from build123d import *

# Parameters (mm, degrees)
SKETCH1_W           = 36.2
SKETCH1_H           = 29.5
BOSS_EXTRUDE1_DEPTH = 5
SKETCH3_W           = 33.053
SKETCH3_H           = 12.372
CUT_EXTRUDE1_DEPTH  = 47.964774033
SKETCH4_W           = 5
SKETCH4_H           = 12.372
BOSS_EXTRUDE2_DEPTH = 3.5
SKETCH5_R           = 14.763665
SKETCH5_R_2         = 12.2036
BOSS_EXTRUDE3_DEPTH = 10


with BuildPart() as part:
    # Sketch1 → Boss-Extrude1 (new body)
    with BuildSketch(Plane.XY):
        with Locations((18.1, 14.75)):
            Rectangle(SKETCH1_W, SKETCH1_H)
    extrude(amount=BOSS_EXTRUDE1_DEPTH)

    # Sketch3 → Cut-Extrude1 (cut, through all)
    with BuildSketch(Plane.XY.offset(5)):
        with Locations((18.1, 14.914)):
            Rectangle(SKETCH3_W, SKETCH3_H)
    extrude(amount=-CUT_EXTRUDE1_DEPTH, mode=Mode.SUBTRACT)

    # Sketch4 → Boss-Extrude2 (add)
    with BuildSketch(Plane.XY.offset(5)):
        with Locations((4.0735, 14.914)):
            Rectangle(SKETCH4_W, SKETCH4_H)
        with Locations((32.1265, 14.914)):
            Rectangle(SKETCH4_W, SKETCH4_H)
    extrude(amount=-BOSS_EXTRUDE2_DEPTH)

    # Sketch5 → Boss-Extrude3 (add)
    with BuildSketch(Plane.XY.offset(5)):
        with Locations(Location((23.79465, 14.75, 0), (0, 0, 204.072563575))):
            Circle(SKETCH5_R)
        with Locations(Location((23.79465, 14.75, 0), (0, 0, 209.568314483))):
            Circle(SKETCH5_R_2, mode=Mode.SUBTRACT)
    extrude(amount=BOSS_EXTRUDE3_DEPTH)


solid = part.part
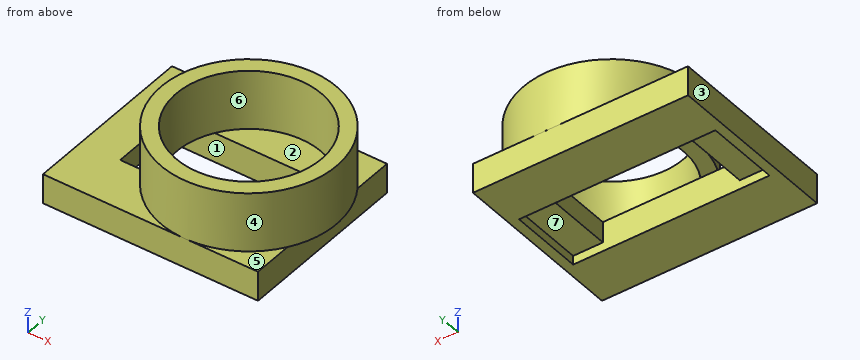
Geometry: final body of the model. Coordinates: model frame, mm. Face numbers are marked on the shaded views. A direction names the side the tool comes from. Give positions to 0.01 mm unless a question says otherwise; leave off trailing zeros. Write each loop counter-clockwise with the first axis right and the second up, starting at its lowest first coordinate (ties: lowest second). Pieces come first, ordered by that corner, then holes. Notation, with made-up numbers: (47.25, 81) - (68.25, 81) arc R20 ccw to (68.25, 104) - close; hole circle Ø9 at (36.5, 17). An arc over 180 degrees is marked (long way). Return JSON: item names as keys, results as strings. Group by question number.
1) Section C-C on y = 7.25. Return the cut outline in (x, z), plus the area to 3 significant figures.
2) First-contact query: P1, Ø3, axis at y = 16.5, z = 4, coming from the +X side; P2, Ø1.3, axis at x = 11.5, y = 12.5, coming from the -Z side; P3, Ø8, axis at y = 15, z = 13, coming from the -X side. Flat tips, straight axial feed; report the tip coordinate or a pass-through.
3) Section D-D on x = 31. Return the cut outline in (y, z).
4) Section B-B on y = 14.75. Return the cut outline in (x, z).
5) Line query: line 1 (X direction, y = 14.75, z = 11.75); line 2 (Y direction, x = 7.5, z = 1.25); line 3 (Y direction, x = 24, z = 13). Output: solid intervals per line, ascending.
6) Mould query, pull axis Y, two halves, no side actions, for the marked faces 1, 2, 3 and 4. Classes: released by +Y, released by -Y, zero draft, split by the parting line, or undercut.
7) Set-up query: the marked faces 5, 6 and 7. Return all of +Z, -Z, +X, -X, +Y, -Y with unobstructed straight access to the full face (end or side cutting, diameter ignored); none if empty.
8) Section A-A on x = 26.5. Return the cut outline in (y, z).
Filled in:
{
 "1": {"outline": "(0, 0) - (36.2, 0) - (36.2, 5) - (36.51, 5) - (36.51, 15) - (33.42, 15) - (33.42, 5) - (14.17, 5) - (14.17, 15) - (11.08, 15) - (11.08, 5) - (0, 5) - close", "area": "243 mm^2"},
 "2": {"P1": "stops at x = 38.54", "P2": "stops at z = 5", "P3": "stops at x = 9.03"},
 "3": {"outline": "(0, 0) - (8.73, 0) - (8.73, 1.5) - (21.1, 1.5) - (21.1, 0) - (29.5, 0) - (29.5, 5) - (27.64, 5) - (27.64, 15) - (24.6, 15) - (24.6, 5) - (4.9, 5) - (4.9, 15) - (1.86, 15) - (1.86, 5) - (0, 5) - close"},
 "4": {"outline": "(0, 0) - (1.57, 0) - (1.57, 1.5) - (6.57, 1.5) - (6.57, 5) - (0, 5) - close; (9.03, 5) - (11.59, 5) - (11.59, 15) - (9.03, 15) - close; (29.63, 1.5) - (34.63, 1.5) - (34.63, 0) - (36.2, 0) - (36.2, 5) - (38.56, 5) - (38.56, 15) - (36, 15) - (36, 5) - (29.63, 5) - close"},
 "5": {"line 1": "x = 9.03 to 11.59, 36 to 38.56", "line 2": "y = 0 to 8.73, 21.1 to 29.5", "line 3": "y = -0.01 to 2.55, 26.95 to 29.51"},
 "6": {"face 1": "undercut", "face 2": "undercut", "face 3": "zero draft", "face 4": "split by the parting line"},
 "7": {"face 5": "+Z, +X, -Y", "face 6": "+Z", "face 7": "-Z"},
 "8": {"outline": "(0, 0) - (8.73, 0) - (8.73, 5) - (2.85, 5) - (2.85, 15) - (0.24, 15) - (0.24, 5) - (0, 5) - close; (21.1, 0) - (29.5, 0) - (29.5, 5) - (29.26, 5) - (29.26, 15) - (26.65, 15) - (26.65, 5) - (21.1, 5) - close"}
}
